Geometry: final body of the model. Coordinates: model frame, mm. Face numbers are marked on the shaded views. Coordinates: 2 decimals unless noted, no trailing zeros. Write each loop counter-clockwise with the first axis right and the second up, starting at its lowest first coordinate (ties: lowest second). Pieces come first, ordered by that corner, then holes. Notation, with made-up numbers: M -21.5,30.25 L -14.5,30.25 A31 ccw -14.5,54.25 Z; hole C 69,79.5 d8. An arc over 180 degrees is marked long. Write item = value, one per line. Start each with the question number.
Item 1: Section B-B on z = 18.5. Output: boundary loops of the cut face in (x, y), plus the area to 3 significant figures.
Item 2: Pull-direction query (X, two-part tool) for the marked faces 1, 2 and 3; classes: +X half, -X half, draft (parallel to the pull), parting line (faces both ways), or undercut.
Item 3: First-contact query: pin 1 Ø2 at (y, z) = (-3.5, 27.5) entering from -X; pin 2 Ø2.5 at (x, y) = (-0.5, -0.5) entering from +Z; pin 3 Ø3 at (x, z) = (-3, 38) entering from +Y. Flat tips, straight axial feed; report the tip coordinate or a pass-through.
Item 4: Section A-A on y = 0. Output: boundary loops of the cut face in (x, z), plus the area to 3 significant figures.
Item 5: Ray query, L1, parallel to X at y = 0.75, z = 38; L2, parallel to Z at x = -1.5, y = 2. Return the intervals inside material, ascending. Write a range as [from, to].
from build123d import *

# Parameters (mm, degrees)
SKETCH_1_W          = 5
SKETCH_1_H          = 6
SKETCH_2_R          = 3
EXTRUDE_1_DEPTH     = 45
CUT_EXTRUDE_1_DEPTH = 4.5
CHAMFER_1_SIZE2     = 0.100043834
CHAMFER_1_SIZE      = 0.100042957
CHAMFER_2_SIZE      = 0.20006968
CHAMFER_2_SIZE2     = 0.200074659


with BuildPart() as part:
    # 草图1 → 旋转1 (revolve)
    with BuildSketch(Plane(origin=(0, 0, 0), x_dir=(1, 0, 0), z_dir=(0, 1, 0))):
        with Locations((2.5, -48)):
            Rectangle(SKETCH_1_W, SKETCH_1_H)
    revolve(axis=Axis((0, 0, 45), (0, 0, 1)))

    # 草图2 → 凸台-拉伸1 (add)
    with BuildSketch(Plane(origin=(0, 0, 45), x_dir=(-1, 0, 0), z_dir=(0, 0, -1))):
        with Locations(Location((0, 0, 0), (0, 0, 180))):
            Circle(SKETCH_2_R)
    extrude(amount=EXTRUDE_1_DEPTH)

    # 草图3 → 切除-拉伸1 (cut)
    with BuildSketch(Plane.XY.offset(51)):
        Polygon((-2.51, -1.449149176), (0, -2.898298351), (2.51, -1.449149176), (2.51, 1.449149176), (0, 2.898298351), (-2.51, 1.449149176), align=None)
    extrude(amount=-CUT_EXTRUDE_1_DEPTH, mode=Mode.SUBTRACT)

    # 倒角1
    chamfer_1_edges = [part.edges().sort_by_distance(p)[0] for p in [
        (-5, 0, 51),
        (-5, 0, 45),
    ]]
    chamfer(chamfer_1_edges, length=CHAMFER_1_SIZE, length2=CHAMFER_1_SIZE2)

    # 倒角2
    chamfer_2_edges = [part.edges().sort_by_distance(p)[0] for p in [
        (-3, 0, 0),
    ]]
    chamfer_2_side = [part.faces().sort_by_distance(p)[0] for p in [
        (-3, 0, 22.5),
    ]]
    chamfer(chamfer_2_edges, length=CHAMFER_2_SIZE, length2=CHAMFER_2_SIZE2, reference=chamfer_2_side[0])


solid = part.part
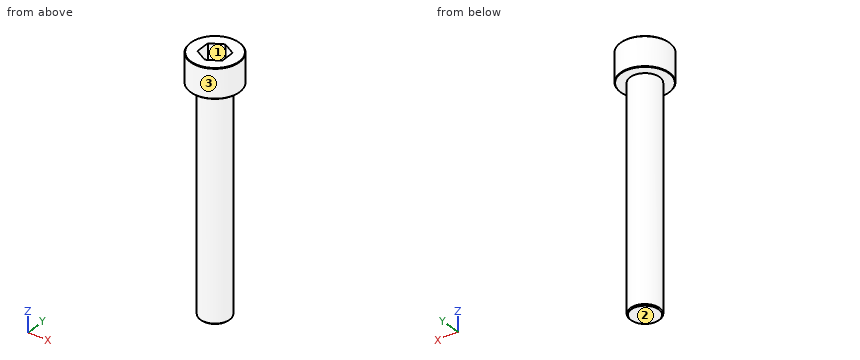
Responses:
q1.outline = C 0,0 d6
q1.area = 28.3 mm²
q2.face_1 = undercut
q2.face_2 = draft
q2.face_3 = parting line
q3.pin_1 = -1.66
q3.pin_2 = 46.5
q3.pin_3 = 2.6
q4.outline = M -5,45.1 L -4.9,45 L -3,45 L -3,0.2 L -2.8,0 L 2.8,0 L 3,0.2 L 3,45 L 4.9,45 L 5,45.1 L 5,50.9 L 4.9,51 L 2.51,51 L 2.51,46.5 L -2.51,46.5 L -2.51,51 L -4.9,51 L -5,50.9 Z
q4.area = 307 mm²
q5.L1 = [-2.9, 2.9]
q5.L2 = [0, 46.5]
